```python
from build123d import *

# Parameters (mm, degrees)
BOSS_EXTRUDE2_DEPTH     = 15
CUT_EXTRUDE3_DEPTH      = 46.552167896
CUT_EXTRUDE3_DEPTH_BACK = 46.552167896
SKETCH4_R               = 2.25


with BuildPart() as part:
    # Sketch1 → Boss-Extrude2 (new body)
    with BuildSketch(Plane.XY):
        with BuildLine():
            ThreePointArc((17.926516672, -2.5), (-1.253006032, -18.056577081), (-18.1, 0))
            Line((-18.1, 0), (-23, 0))
            Line((-23, 0), (-35, 0))
            Line((-35, 0), (-35, -22.5))
            Line((-35, -22.5), (-35, -25))
            Line((-35, -25), (35, -25))
            Line((35, -25), (35, -22.5))
            Line((35, -22.5), (35, -7.5))
            Line((35, -7.5), (35, -2.5))
            Line((35, -2.5), (17.926516672, -2.5))
        make_face()
        with BuildLine():
            Line((17.926516672, 2.5), (35, 2.5))
            Line((35, 2.5), (35, 7.5))
            Line((35, 7.5), (21.742814905, 7.5))
            ThreePointArc((21.742814905, 7.5), (-3.802318844, 22.683526432), (-23, 0))
            Line((-23, 0), (-18.1, 0))
            ThreePointArc((-18.1, 0), (-1.253006032, 18.056577081), (17.926516672, 2.5))
        make_face()
    extrude(amount=BOSS_EXTRUDE2_DEPTH)

    # Sketch4 → Cut-Extrude3 (cut, two sides: drawn at the far end of the back side and taken through both)
    with BuildSketch(Plane(origin=(0, 0, 0), x_dir=(1, 0, 0), z_dir=(0, 1, 0)).offset(-CUT_EXTRUDE3_DEPTH_BACK)):
        with Locations(Location((-28.75, -7.5, 0), (0, 0, 180))):
            Circle(SKETCH4_R)
        with Locations(Location((28.75, -7.5, 0), (0, 0, 180))):
            Circle(SKETCH4_R)
    extrude(amount=CUT_EXTRUDE3_DEPTH + CUT_EXTRUDE3_DEPTH_BACK, mode=Mode.SUBTRACT)


solid = part.part
```
Here's how the part is built. I have some questions about the finished solid (model axes, mm). A direction names the side the tool comes from. Give positions to 0.01 mm unless a question says otherwise; leave off trailing zeros. Write each loop counter-clockwise with the first axis right and the second up, starting at its lowest first coordinate (ties: lowest second). Pieces come first, ordered by that corner, then holes. Notation, with made-up numbers: (54, 9.5) -> (83, 9.5) arc R29 cw to (83, 35.5) -> close; hole circle Ø11 at (22.5, 81.5). An arc over 180 degrees is marked (long way). Write each question's results on one line, items separated by ' | '.
Item 1: Suppose I cut it at B-B on x = 0. Write out the boundary of the cut face in (y, z), plus the area to 3 significant figures.
Output:
outline: (-25, 0) -> (-18.1, 0) -> (-18.1, 15) -> (-25, 15) -> close; (18.1, 0) -> (23, 0) -> (23, 15) -> (18.1, 15) -> close | area: 177 mm^2
Item 2: Suppose I cut it at C-C on y = -17. Write out the boundary of the cut face in (x, z), plus the area to 3 significant figures.
Output:
outline: (-35, 0) -> (-6.21, 0) -> (-6.21, 15) -> (-35, 15) -> close; (6.21, 0) -> (35, 0) -> (35, 15) -> (6.21, 15) -> close; hole circle Ø4.5 at (-28.75, 7.5); hole circle Ø4.5 at (28.75, 7.5) | area: 832 mm^2
Item 3: Suppose I cut it at D-D on z = 11. Write out the boundary of the cut face in (x, y), plus the area to 3 significant figures.
Output:
outline: (-35, -25) -> (35, -25) -> (35, -2.5) -> (17.93, -2.5) arc R18.1 cw (long way) to (17.93, 2.5) -> (35, 2.5) -> (35, 7.5) -> (21.74, 7.5) arc R23 ccw to (-23, 0) -> (-35, 0) -> close | area: 1,560 mm^2
Item 4: Suppose I cut it at A-A on z = 7.5. Write out the boundary of the cut face in (x, y).
Output:
outline: (-35, -25) -> (-31, -25) -> (-31, 0) -> (-35, 0) -> close; (-26.5, -25) -> (26.5, -25) -> (26.5, -2.5) -> (17.93, -2.5) arc R18.1 cw (long way) to (17.93, 2.5) -> (26.5, 2.5) -> (26.5, 7.5) -> (21.74, 7.5) arc R23 ccw to (-23, 0) -> (-26.5, 0) -> close; (31, -25) -> (35, -25) -> (35, -2.5) -> (31, -2.5) -> close; (31, 2.5) -> (35, 2.5) -> (35, 7.5) -> (31, 7.5) -> close
Item 5: If I drill on L1, parallel to X at y = -19.5, z = 7.5; L2, parallel to X at y = -13, z = 7.5; L3, parallel to X at y = -18.5, z = 5.5, over which ranges is the centre line in solid material (lowest first)?
Output:
L1: x = -35 to -31, -26.5 to 26.5, 31 to 35 | L2: x = -35 to -31, -26.5 to -12.59, 12.59 to 26.5, 31 to 35 | L3: x = -35 to -29.78, -27.72 to 27.72, 29.78 to 35
Item 6: We'd pull the mould along Z, two halves only. Please class faces 4 (the face through (26.604, 4.965, 8.176)), 5 (the face through (-32, 0, 7)), 6 (the face through (-8, -17, 0)): pulls with the +Z half, pulls with the -Z half, needs draft (parallel to the pull), parting line crosses it, or undercut.
Output:
face 4: undercut | face 5: needs draft | face 6: pulls with the -Z half
Item 7: On a 3-axis mill with a long thin cutter (end or side, diameter ignored), from which of +Z, -Z, +X, -X, +Y, -Y can I reach the whole of each face in a straight line? I mean faces 1 (the face through (26, 2.5, 7)), 2 (the face through (-30.896, -12.675, 8.176)), 3 (the face through (27, 7.5, 5.7)). Say none if no direction works.
Output:
face 1: +Z, -Z, +X | face 2: +Y, -Y | face 3: +Z, -Z, +X, +Y
Item 8: For pin 1 Ø7.5 at (x, z) = (23.5, 8) entering from +Y; pin 2 Ø6.5 at (x, z) = (28.5, 4.5) entering from +Y, each with a flat end and sliding along its axis, tell me the tip position at first contact or that it passes through.
Output:
pin 1: stops at y = 11.79 | pin 2: stops at y = 7.5
